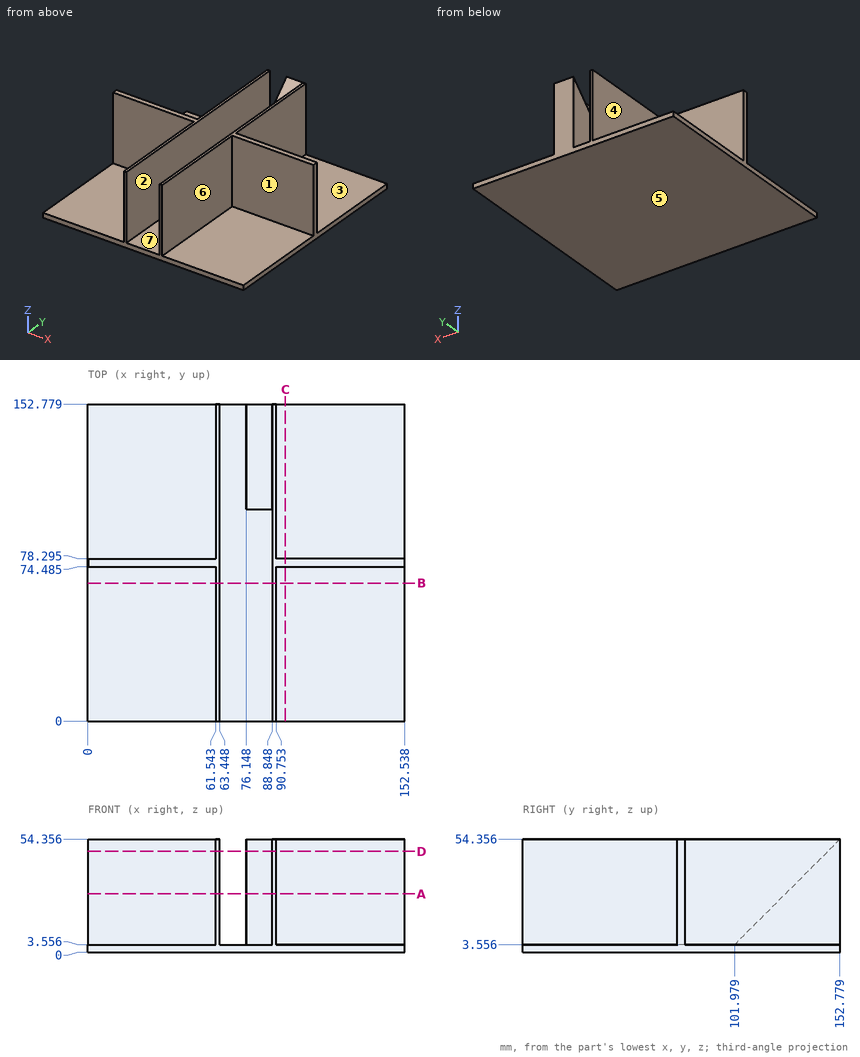
Geometry: see drawing. Coordinates: mm, zero at the bounding-box minimum. A direction names the side the tool comes from. Give positions to 0.01 mm unless a question says otherwise; leave off trailing zeros. Order: outer loops, then holes, each group sorted by start corner. A loop starts at its lowest first (then second) coordinate and runs counter-clockwise, first axis right, second up. Notation, with made-up numbers: (-29, 46.25) - (-13, 46.25) arc R13 ccw to (-13, 59.25) - close; hole circle Ø11 at (-29.5, 73). An arc over 180 degrees is marked (long way). Write each question's results on one line, items separated by ' | '.
Item 1: Section A-A (z = 28). Return loops of the section in (x, y) (1 decimal), and give its area (3 significant figures).
A:
outline: (0, 74.5) - (61.5, 74.5) - (61.5, 0) - (63.4, 0) - (63.4, 152.8) - (61.5, 152.8) - (61.5, 78.3) - (0, 78.3) - close; (76.1, 126.4) - (88.8, 126.4) - (88.8, 0) - (90.8, 0) - (90.8, 74.5) - (152.5, 74.5) - (152.5, 78.3) - (90.8, 78.3) - (90.8, 152.8) - (76.1, 152.8) - close | area: 1,390 mm^2
Item 2: Access query for the marked faces 1, 2 and 3. Directions: +Z, -Z, +X, -X, +Y, -Y. A direction counts if a zero-diameter tool reaches every point of the face in a straight line with its end or side. Return the directions, or none.
A:
face 1: +Z, +X, -Y | face 2: +Z, +Y, -Y | face 3: +Z, +X, +Y
Item 3: Section B-B (y = 66.5). Return loops of the section in (x, z), and give its area (3 significant figures).
A:
outline: (0, 0) - (152.54, 0) - (152.54, 3.56) - (90.75, 3.56) - (90.75, 54.36) - (88.85, 54.36) - (88.85, 3.56) - (63.45, 3.56) - (63.45, 54.36) - (61.54, 54.36) - (61.54, 3.56) - (0, 3.56) - close | area: 736 mm^2
Item 4: Contact query for flat-ended pins moving along their axis: pin 1 Ø2 at (y, z) = (136.5, 29.5) entering from +X; pin 2 Ø8 at (x, z) = (123, 13.5) entering from -Y (1 decimal); pin 3 Ø6 at (x, z) = (82.5, 49) entering from -Y. Output: stop coordinate, or through.
A:
pin 1: stops at x = 90.75 | pin 2: stops at y = 74.5 | pin 3: stops at y = 144.42
Item 5: Material intervals for line 1 along X through (y, z) = (121.5, 8.5); line 2 along X through (y, z) = (21, 24); line 3 along Z through (x, y) = (18.5, 85.5), sorted ascending.
A:
line 1: x = 61.54 to 63.45, 76.15 to 90.75 | line 2: x = 61.54 to 63.45, 88.85 to 90.75 | line 3: z = 0 to 3.56
Item 6: Section D-D (z = 48.5). Return loops of the section in (x, y) (1 decimal), and give its area (3 significant figures).
A:
outline: (0, 74.5) - (61.5, 74.5) - (61.5, 0) - (63.4, 0) - (63.4, 152.8) - (61.5, 152.8) - (61.5, 78.3) - (0, 78.3) - close; (76.1, 146.9) - (88.8, 146.9) - (88.8, 0) - (90.8, 0) - (90.8, 74.5) - (152.5, 74.5) - (152.5, 78.3) - (90.8, 78.3) - (90.8, 152.8) - (76.1, 152.8) - close | area: 1,130 mm^2
Item 7: Draft query along X for the marked faces 4, 5, 6 and 7. Return one class per face: released by +X, released by -X, zero draft, split by the parting line, or undercut.
A:
face 4: released by -X | face 5: zero draft | face 6: released by +X | face 7: undercut
Item 8: Section C-C (x = 95). Return loops of the section in (y, z) (1 decimal), and give its area (3 significant figures).
A:
outline: (0, 0) - (152.8, 0) - (152.8, 3.6) - (78.3, 3.6) - (78.3, 54.4) - (74.5, 54.4) - (74.5, 3.6) - (0, 3.6) - close | area: 737 mm^2
